Source: CAD feature listing. Evaluate the final solid. Frame: model axes, mm. A direction names the side the tool comes from. Round coordinates to 2 decimals unless told otherwise and drop trailing zeros. Order: outer loops, then holes, each group sorted by start corner. A loop starts at its lowest first (then second) coordinate and runs counter-clockwise, first axis right, second up. Notation, with made-up numbers: (32.25, 62) -> (48.25, 62) arc R21 ccw to (48.25, 94) -> close; hole circle Ø1 at (14, 78). An arc over 180 degrees is marked (long way). Answer as CSV lines item,"result".
from build123d import *

# Parameters (mm, degrees)
SKETCH_1_W          = 37
SKETCH_1_H          = 5
EXTRUDE_1_DEPTH     = 19
SKETCH_2_R          = 18.5
EXTRUDE_2_DEPTH     = 5
SKETCH_3_R          = 6
SKETCH_3_R_2        = 1.5
CUT_EXTRUDE_1_DEPTH = 5
M3X0_5_1_D          = 2.5
M3X0_5_1_DEPTH      = 10
M3X0_5_1_TIP        = 0.751075774


with BuildPart() as part:
    # ｽｹｯﾁ1 → ﾎﾞｽ - 押し出し1 (new body)
    with BuildSketch(Plane.XY):
        Rectangle(SKETCH_1_W, SKETCH_1_H)
    extrude(amount=EXTRUDE_1_DEPTH)

    # ｽｹｯﾁ2 → ﾎﾞｽ - 押し出し2 (add)
    with BuildSketch(Plane.XZ.offset(2.5)):
        with Locations((0, 19)):
            Circle(SKETCH_2_R)
    extrude(amount=-EXTRUDE_2_DEPTH)

    # ｽｹｯﾁ3 → ｶｯﾄ - 押し出し1 (cut)
    with BuildSketch(Plane.XZ.offset(2.5)):
        with Locations(Location((0, 26, 0), (0, 0, 270))):  # turned: the seam where the file's is
            Circle(SKETCH_3_R)
        with Locations(Location((-15.5, 19, 0), (0, 0, 270))):  # turned: the seam where the file's is
            Circle(SKETCH_3_R_2)
        with Locations(Location((7.75, 5.576606241, 0), (0, 0, 270))):  # turned: the seam where the file's is
            Circle(SKETCH_3_R_2)
        with Locations(Location((7.75, 32.423393759, 0), (0, 0, 270))):  # turned: the seam where the file's is
            Circle(SKETCH_3_R_2)
    extrude(amount=-CUT_EXTRUDE_1_DEPTH, mode=Mode.SUBTRACT)

    # M3x0.5 ねじ穴1
    with Locations(Plane(origin=(0, 0, 0), x_dir=(-1, 0, 0), z_dir=(0, 0, -1))):
        with Locations((15, 0), (-15, 0)):
            Hole(M3X0_5_1_D / 2, depth=M3X0_5_1_DEPTH)
            with Locations((0, 0, -(M3X0_5_1_DEPTH + M3X0_5_1_TIP / 2))):  # 118° drill point
                Cone(0, M3X0_5_1_D / 2, M3X0_5_1_TIP, mode=Mode.SUBTRACT)


solid = part.part
1. Section query B-B on x = 7.75. Return loops of the section in (y, z).
Results below:
outline,"(-2.5, 0) -> (2.5, 0) -> (2.5, 4.08) -> (-2.5, 4.08) -> close; (-2.5, 7.08) -> (2.5, 7.08) -> (2.5, 30.92) -> (-2.5, 30.92) -> close; (-2.5, 33.92) -> (2.5, 33.92) -> (2.5, 35.8) -> (-2.5, 35.8) -> close"
2. Section query A-A on z = 9. Return loops of the section in (x, y).
Results below:
outline,"(-18.5, -2.5) -> (18.5, -2.5) -> (18.5, 2.5) -> (-18.5, 2.5) -> close; hole circle Ø2.5 at (-15, 0); hole circle Ø2.5 at (15, 0)"
3. Section query C-C on z = 18.5. Return loops of the section in (x, y).
Results below:
outline,"(-18.5, -2.5) -> (-16.91, -2.5) -> (-16.91, 2.5) -> (-18.5, 2.5) -> close; (-14.09, -2.5) -> (18.5, -2.5) -> (18.5, 2.5) -> (-14.09, 2.5) -> close"
4. Reachability of faces 1 (the flat face through (0, 2.5, 15)), 2 (the cylindrical face through (-16.25, 0.05, 5.07)) from +Z, -Z, +X, -X, +Y, -Y: full face, straight path, thin tool, end or side. Return the list, or none.
Results below:
face 1,"+Z, -Z, +X, -X, +Y"
face 2,"-Z"
5. Section query D-D on x = -4.5. Return loops of the section in (y, z), and give its area (3 significant figures).
Results below:
outline,"(-2.5, 0) -> (2.5, 0) -> (2.5, 22.03) -> (-2.5, 22.03) -> close; (-2.5, 29.97) -> (2.5, 29.97) -> (2.5, 36.94) -> (-2.5, 36.94) -> close"
area,"145 mm2"
6. Line query: L1, parallel to X at y = 0.25, z = 2; L2, parallel to Z at x = 6.5, y = -0.5; L3, parallel to Z at x = -15, y = -1.85. Output: solid intervals per line, ascending. Write a range as [from, to].
Results below:
L1,"[-18.5, -16.22], [-13.78, 13.78], [16.22, 18.5]"
L2,"[0, 4.75], [6.41, 31.59], [33.25, 36.32]"
L3,"[0, 17.59], [20.41, 29.83]"
7. Mould query, pull axis X, two halves, no side actions, for faces 3 (the cylindrical face through (0.407, -0.035, 37.496)), 4 (the cylindrical face through (13.75, 0.05, 5.07)), 5 (the flat face through (0, 0, 0)), 6 (the cylindrical face through (-15.43, -0.04, 20.5)). Classes: released by +X, released by -X, zero draft, split by the parting line, or undercut.
Results below:
face 3,"split by the parting line"
face 4,"undercut"
face 5,"zero draft"
face 6,"undercut"
8. Pin query (flat end, axial travel): pin 1 (2 mm diameter, centred on x = 15, y = 0, fed in from +Z); pin 2 (1.5 mm diameter, centred on x = -11.5, y = -1, fed in from +Z); pin 3 (3 mm diameter, centred on x = 14.5, y = -0.5, fed in from +Z). Return the tip coordinate at first contact, or that it passes through.
Results below:
pin 1,"z = 31.09"
pin 2,"z = 34.06"
pin 3,"z = 32.16"
